Answer from the drawing. Dimensions are ordinates in mm from the lowest x, y and z of the part. Coordinates: 2 decimals unless noted, no trailing zeros. Order: outer loops, then holes, each group sorted by start corner. A loop starts at its lowest first (then second) coordinate and runs counter-clockwise, first axis right, second up.
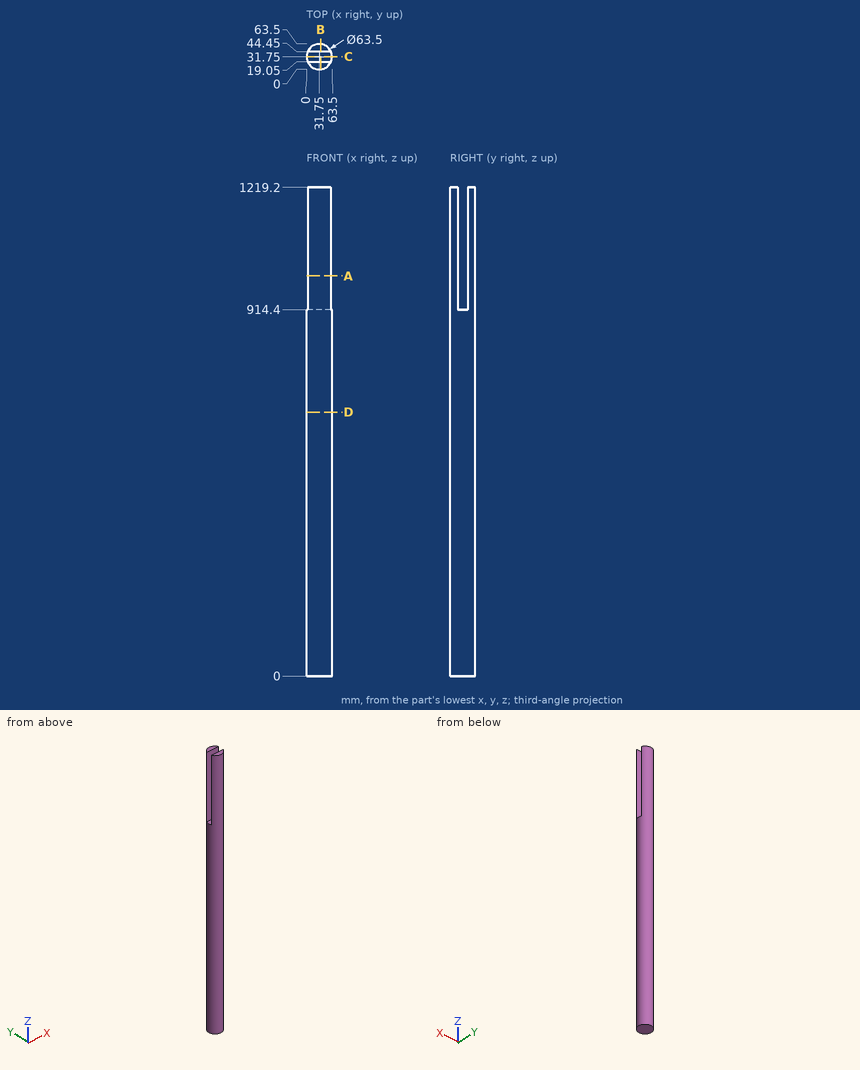
1. The part is cut by section A-A (z = 998.5). Determine the outline of the cut face in (x, y).
2. The part is cut by section B-B (x = 35). Determine the outline of the cut face in (y, z).
3. The part is cut by section C-C (y = 31.75). Determine the outline of the cut face in (x, z), plus the area to 3 significant figures.
4. The part is cut by section D-D (z = 658.5). Determine the outline of the cut face in (x, y).
5. Flat-ended cylindrical pins translate along their axes: pin 1 (6 mm diameter, centred on x = 20.5, z = 409, fed in from -Y); pin 2 (2 mm diameter, centred on x = 48.5, z = 705, fed in from -Y); pin 3 (1 mm diameter, centred on y = 12.5, z = 315.5, fed in from +X). Find the tip coordinate at first contact, or state that the pin passes through.
6. Consider probe 1 along Y at (x, z) = (19, 1117.5); probe 2 along X at (y, z) = (19, 238); probe 3 along Z at (x, y) = (57, 30.5). Determine where each line is inside the solid, lowest interval first.
Worked out:
1. outline: (2.65, 19.05) arc R31.75 ccw to (60.85, 19.05) - close; (2.65, 44.45) - (60.85, 44.45) arc R31.75 ccw to start
2. outline: (0.17, 0) - (63.33, 0) - (63.33, 1219.2) - (44.45, 1219.2) - (44.45, 914.4) - (19.05, 914.4) - (19.05, 1219.2) - (0.17, 1219.2) - close
3. outline: (0, 0) - (63.5, 0) - (63.5, 914.4) - (0, 914.4) - close
3. area: 58,100 mm2
4. outline: circle Ø63.5 at (31.75, 31.75)
5. pin 1: stops at y = 1.09
5. pin 2: stops at y = 4.18
5. pin 3: stops at x = 57.37
6. probe 1: y = 2.67 to 19.05, 44.45 to 60.83
6. probe 2: x = 2.67 to 60.83
6. probe 3: z = 0 to 914.4
